from build123d import *

# Parameters (mm, degrees)
F1_DEPTH  = 330.2
F2_W      = 165.1
F2_H      = 35.56
F3_DEPTH  = 228.6
F4_SIZE   = 3.81
F6_DEPTH  = 25.4
F8_DEPTH  = 0.635
F9_DEPTH  = 25.4
F10_R     = 15.875
F11_DEPTH = 25.4
F12_SIZE  = 0.635


with BuildPart() as f1:
    # F0 (on Front) → F1 (new body)
    with BuildSketch(Plane.XZ):
        with BuildLine():
            Line((-76.581, 48.895), (-76.581, 0))
            Line((-76.581, 0), (76.581, 0))
            Line((76.581, 0), (76.581, 48.895))
            ThreePointArc((76.581, 48.895), (75.6510640303, 51.1400640303), (73.406, 52.07))
            Line((73.406, 52.07), (72.895141329, 52.07))
            ThreePointArc((72.895141329, 52.07), (70.8542906682, 51.3271911069), (69.7683767132, 49.4463329641))
            Line((69.7683767132, 49.4463329641), (63.3185122812, 12.8673340718))
            ThreePointArc((63.3185122812, 12.8673340718), (61.146684371, 9.1056177862), (57.0649830495, 7.62))
            Line((57.0649830495, 7.62), (0, 7.62))
            Line((0, 7.62), (-57.0649830495, 7.62))
            ThreePointArc((-57.0649830495, 7.62), (-61.146684371, 9.1056177862), (-63.3185122812, 12.8673340718))
            Line((-63.3185122812, 12.8673340718), (-69.7683767132, 49.4463329641))
            ThreePointArc((-69.7683767132, 49.4463329641), (-70.8542906682, 51.3271911069), (-72.895141329, 52.07))
            Line((-72.895141329, 52.07), (-73.406, 52.07))
            ThreePointArc((-73.406, 52.07), (-75.6510640303, 51.1400640303), (-76.581, 48.895))
        make_face()
    extrude(amount=F1_DEPTH)

    # F2 (on face) → F3 (cut)
    with BuildSketch(Plane.XZ.offset(330.2)):
        with Locations((0, 39.37)):
            Rectangle(F2_W, F2_H)
    extrude(amount=-F3_DEPTH, mode=Mode.SUBTRACT)

    # F4
    f4_edges = [f1.edges().sort_by_distance(p)[0] for p in [
        (76.581, -215.9, 21.59),
        (-76.581, -215.9, 21.59),
    ]]
    chamfer(f4_edges, length=F4_SIZE)

    # F5 (on face) → F6 (cut)
    with BuildSketch(Plane.XY.offset(7.62)):
        with BuildLine():
            Line((-57.9536338645, -28.1246478687), (-42.1049536604, -43.9733280728))
            ThreePointArc((-42.1049536604, -43.9733280728), (-53.0225, -76.2), (-42.1049536604, -108.4266719272))
            Line((-42.1049536604, -108.4266719272), (-57.9536338645, -124.2753521313))
            ThreePointArc((-57.9536338645, -124.2753521313), (-57.9536338645, -134.1536338645), (-48.0753521313, -134.1536338645))
            Line((-48.0753521313, -134.1536338645), (-32.2266719272, -118.3049536604))
            ThreePointArc((-32.2266719272, -118.3049536604), (0, -129.2225), (32.2266719272, -118.3049536604))
            Line((32.2266719272, -118.3049536604), (48.0753521313, -134.1536338645))
            ThreePointArc((48.0753521313, -134.1536338645), (57.9536338645, -134.1536338645), (57.9536338645, -124.2753521313))
            Line((57.9536338645, -124.2753521313), (42.1049536604, -108.4266719272))
            ThreePointArc((42.1049536604, -108.4266719272), (53.0225, -76.2), (42.1049536604, -43.9733280728))
            Line((42.1049536604, -43.9733280728), (57.9536338645, -28.1246478687))
            ThreePointArc((57.9536338645, -28.1246478687), (57.9536338645, -18.2463661355), (48.0753521313, -18.2463661355))
            Line((48.0753521313, -18.2463661355), (32.2266719272, -34.0950463396))
            ThreePointArc((32.2266719272, -34.0950463396), (0, -23.1775), (-32.2266719272, -34.0950463396))
            Line((-32.2266719272, -34.0950463396), (-48.0753521313, -18.2463661355))
            ThreePointArc((-48.0753521313, -18.2463661355), (-57.9536338645, -18.2463661355), (-57.9536338645, -28.1246478687))
        make_face()
    extrude(amount=-F6_DEPTH, mode=Mode.SUBTRACT)

    # F7 (on face) → F8 (cut)
    with BuildSketch(Plane.XY.offset(7.62)):
        with BuildLine():
            ThreePointArc((-60.1986978948, -30.3697118989), (-49.1264293251, -32.5721230524), (-42.8544929979, -23.1855070021))
            ThreePointArc((-42.8544929979, -23.1855070021), (-43.6278769476, -19.2974433292), (-45.8302881011, -16.0013021052))
            ThreePointArc((-45.8302881011, -16.0013021052), (-60.1986978948, -16.0013021052), (-60.1986978948, -30.3697118989))
        make_face()
        with BuildLine():
            ThreePointArc((-45.8302881011, -16.0013021052), (-43.6278769476, -19.2974433292), (-42.8544929979, -23.1855070021))
            ThreePointArc((-42.8544929979, -23.1855070021), (-49.1264293251, -32.5721230524), (-60.1986978948, -30.3697118989))
            Line((-60.1986978948, -30.3697118989), (-43.1340409794, -47.4343688143))
            Line((-43.1340409794, -47.4343688143), (-28.767801471, -33.0637887353))
            Line((-28.767801471, -33.0637887353), (-45.8302881011, -16.0013021052))
        make_face()
        with BuildLine():
            ThreePointArc((-45.8302881011, -136.3986978948), (-43.6278769476, -133.1025566708), (-42.8544929979, -129.2144929979))
            ThreePointArc((-42.8544929979, -129.2144929979), (-49.1264293251, -119.8278769476), (-60.1986978948, -122.0302881011))
            ThreePointArc((-60.1986978948, -122.0302881011), (-60.1986978948, -136.3986978948), (-45.8302881011, -136.3986978948))
        make_face()
        with BuildLine():
            ThreePointArc((-60.1986978948, -122.0302881011), (-49.1264293251, -119.8278769476), (-42.8544929979, -129.2144929979))
            ThreePointArc((-42.8544929979, -129.2144929979), (-43.6278769476, -133.1025566708), (-45.8302881011, -136.3986978948))
            Line((-45.8302881011, -136.3986978948), (-28.7656311857, -119.3340409794))
            Line((-28.7656311857, -119.3340409794), (-43.1362112647, -104.967801471))
            Line((-43.1362112647, -104.967801471), (-60.1986978948, -122.0302881011))
        make_face()
        with BuildLine():
            ThreePointArc((45.8302881011, -136.3986978948), (56.9025566708, -138.6011090482), (63.1744929979, -129.2144929979))
            ThreePointArc((63.1744929979, -129.2144929979), (62.4011090482, -125.3264293251), (60.1986978948, -122.0302881011))
            ThreePointArc((60.1986978948, -122.0302881011), (45.8302881011, -122.0302881011), (45.8302881011, -136.3986978948))
        make_face()
        with BuildLine():
            ThreePointArc((45.8302881011, -136.3986978948), (45.8302881011, -122.0302881011), (60.1986978948, -122.0302881011))
            Line((60.1986978948, -122.0302881011), (43.1340409794, -104.9656311857))
            Line((43.1340409794, -104.9656311857), (28.767801471, -119.3362112647))
            Line((28.767801471, -119.3362112647), (45.8302881011, -136.3986978948))
        make_face()
        with BuildLine():
            ThreePointArc((60.1986978948, -30.3697118989), (62.4011090482, -27.0735706749), (63.1744929979, -23.1855070021))
            ThreePointArc((63.1744929979, -23.1855070021), (56.9025566708, -13.7988909518), (45.8302881011, -16.0013021052))
            ThreePointArc((45.8302881011, -16.0013021052), (45.8302881011, -30.3697118989), (60.1986978948, -30.3697118989))
        make_face()
        with BuildLine():
            ThreePointArc((60.1986978948, -30.3697118989), (45.8302881011, -30.3697118989), (45.8302881011, -16.0013021052))
            Line((45.8302881011, -16.0013021052), (28.7656311857, -33.0659590206))
            Line((28.7656311857, -33.0659590206), (43.1362112647, -47.432198529))
            Line((43.1362112647, -47.432198529), (60.1986978948, -30.3697118989))
        make_face()
    extrude(amount=-F8_DEPTH, mode=Mode.SUBTRACT)

    # F7 (on face) → F9 (cut)
    with BuildSketch(Plane.XY.offset(7.62)):
        with BuildLine():
            ThreePointArc((-60.1986978948, -30.3697118989), (-49.1264293251, -32.5721230524), (-42.8544929979, -23.1855070021))
            ThreePointArc((-42.8544929979, -23.1855070021), (-43.6278769476, -19.2974433292), (-45.8302881011, -16.0013021052))
            ThreePointArc((-45.8302881011, -16.0013021052), (-60.1986978948, -16.0013021052), (-60.1986978948, -30.3697118989))
        make_face()
        with BuildLine():
            ThreePointArc((-45.8302881011, -16.0013021052), (-43.6278769476, -19.2974433292), (-42.8544929979, -23.1855070021))
            ThreePointArc((-42.8544929979, -23.1855070021), (-49.1264293251, -32.5721230524), (-60.1986978948, -30.3697118989))
            Line((-60.1986978948, -30.3697118989), (-43.1340409794, -47.4343688143))
            Line((-43.1340409794, -47.4343688143), (-28.767801471, -33.0637887353))
            Line((-28.767801471, -33.0637887353), (-45.8302881011, -16.0013021052))
        make_face()
        with BuildLine():
            ThreePointArc((-45.8302881011, -136.3986978948), (-43.6278769476, -133.1025566708), (-42.8544929979, -129.2144929979))
            ThreePointArc((-42.8544929979, -129.2144929979), (-49.1264293251, -119.8278769476), (-60.1986978948, -122.0302881011))
            ThreePointArc((-60.1986978948, -122.0302881011), (-60.1986978948, -136.3986978948), (-45.8302881011, -136.3986978948))
        make_face()
        with BuildLine():
            ThreePointArc((-60.1986978948, -122.0302881011), (-49.1264293251, -119.8278769476), (-42.8544929979, -129.2144929979))
            ThreePointArc((-42.8544929979, -129.2144929979), (-43.6278769476, -133.1025566708), (-45.8302881011, -136.3986978948))
            Line((-45.8302881011, -136.3986978948), (-28.7656311857, -119.3340409794))
            Line((-28.7656311857, -119.3340409794), (-43.1362112647, -104.967801471))
            Line((-43.1362112647, -104.967801471), (-60.1986978948, -122.0302881011))
        make_face()
        with BuildLine():
            ThreePointArc((45.8302881011, -136.3986978948), (56.9025566708, -138.6011090482), (63.1744929979, -129.2144929979))
            ThreePointArc((63.1744929979, -129.2144929979), (62.4011090482, -125.3264293251), (60.1986978948, -122.0302881011))
            ThreePointArc((60.1986978948, -122.0302881011), (45.8302881011, -122.0302881011), (45.8302881011, -136.3986978948))
        make_face()
        with BuildLine():
            ThreePointArc((45.8302881011, -136.3986978948), (45.8302881011, -122.0302881011), (60.1986978948, -122.0302881011))
            Line((60.1986978948, -122.0302881011), (43.1340409794, -104.9656311857))
            Line((43.1340409794, -104.9656311857), (28.767801471, -119.3362112647))
            Line((28.767801471, -119.3362112647), (45.8302881011, -136.3986978948))
        make_face()
        with BuildLine():
            ThreePointArc((60.1986978948, -30.3697118989), (62.4011090482, -27.0735706749), (63.1744929979, -23.1855070021))
            ThreePointArc((63.1744929979, -23.1855070021), (56.9025566708, -13.7988909518), (45.8302881011, -16.0013021052))
            ThreePointArc((45.8302881011, -16.0013021052), (45.8302881011, -30.3697118989), (60.1986978948, -30.3697118989))
        make_face()
        with BuildLine():
            ThreePointArc((60.1986978948, -30.3697118989), (45.8302881011, -30.3697118989), (45.8302881011, -16.0013021052))
            Line((45.8302881011, -16.0013021052), (28.7656311857, -33.0659590206))
            Line((28.7656311857, -33.0659590206), (43.1362112647, -47.432198529))
            Line((43.1362112647, -47.432198529), (60.1986978948, -30.3697118989))
        make_face()
    extrude(amount=F9_DEPTH, mode=Mode.SUBTRACT)

    # F10 (on face) → F11 (cut)
    with BuildSketch(Plane(origin=(0, 0, 0), x_dir=(1, 0, 0), z_dir=(0, 0, -1))):
        with Locations((0, 285.75)):
            Circle(F10_R)
        with Locations((0, 203.2)):
            Circle(F10_R)
    extrude(amount=-F11_DEPTH, mode=Mode.SUBTRACT)

    # F12
    f12_edges = [f1.edges().sort_by_distance(p)[0] for p in [
        (-15.875, -203.2, 7.62),
        (-15.875, -203.2, 0),
        (-15.875, -285.75, 0),
        (-15.875, -285.75, 7.62),
    ]]
    chamfer(f12_edges, length=F12_SIZE)


solid = f1.part
CAD build for the part. Positions are in the model's coordinates, mm. A direction names the side the tool comes from. Coordinates: 2 decimals unless noted, no trailing zeros. Order: outer loops, then holes, each group sorted by start corner. A loop starts at its lowest first (then second) coordinate and runs counter-clockwise, first axis right, second up. Notation, with made-up numbers: (-24.75, 42.25) -> (24.25, 42.25) arc R14 cw to (24.25, 56.25) -> close; hole circle Ø9 at (-0.5, 37). An arc over 180 degrees is marked (long way). Answer in a Markdown table with one row per item.
1) Drill centre lines: line 1 (X direction, y = -203, z = 3); line 2 (X direction, y = -144, z = 13); line 3 (Z direction, x = -1, y = -225). Where is each one in solid material? Low to high.
Check values:
| item | result |
|---|---|
| line 1 | -76.58 to -15.87, 15.87 to 76.58 |
| line 2 | -76.58 to -63.34, 63.34 to 76.58 |
| line 3 | 0 to 7.62 |
2) Which spindle directions (+Z, -Z, +X, -X, +Y, -Y) get a long thin tool onto all of the face, cutting with end or side? Do faces 1 (the face through (-63.153, -129.877, 8.408)), 2 (the face through (0.48, -23.18, 3.86)), 3 (the face through (-61.099, -162.789, 9.066)). Say none if no direction does.
Check values:
| item | result |
|---|---|
| face 1 | +Z |
| face 2 | +Z, -Z |
| face 3 | +Z, +Y, -Y |
3) Flat gauge pins, fed straight in: P1, Ø17, axis at x = 47.5, y = -125, coming from the +Z side (3 decimals); P2, Ø12, axis at x = 53.5, y = -123, coming from the +Z side; P3, Ø13, axis at x = -68.5, z = 37.5, coming from the -Y side. Where does each tip first touch, or does it go through?
Check values:
| item | result |
|---|---|
| P1 | z = 6.985 |
| P2 | z = 7.97 |
| P3 | y = -101.6 |
4) Band-saw the part on B-B (y = -203.2). List the corners of the cut face in (x, z) (3 decimals), and give its area (3 significant figures).
Check values:
| item | result |
|---|---|
| outline | (-76.581, 0) -> (-16.51, 0) -> (-15.875, 0.635) -> (-15.875, 6.985) -> (-16.51, 7.62) -> (-57.065, 7.62) arc R6.35 cw to (-63.319, 12.867) -> (-64.857, 21.59) -> (-72.771, 21.59) -> (-76.581, 17.78) -> close; (15.875, 0.635) -> (16.51, 0) -> (76.581, 0) -> (76.581, 17.78) -> (72.771, 21.59) -> (64.857, 21.59) -> (63.319, 12.867) arc R6.35 cw to (57.065, 7.62) -> (16.51, 7.62) -> (15.875, 6.985) -> close |
| area | 1,280 mm2 |
5) Band-saw the part on C-C (z = 42.5). List the corners of the cut face in (x, y), and give its area (3 significant figures).
Check values:
| item | result |
|---|---|
| outline | (-76.58, -101.6) -> (-68.54, -101.6) -> (-68.54, 0) -> (-76.58, 0) -> close; (68.54, -101.6) -> (76.58, -101.6) -> (76.58, 0) -> (68.54, 0) -> close |
| area | 1,630 mm2 |
6) Band-saw the part on A-A (x = 0). List the corners of the cut face in (y, z) (1 decimal), and give its area (3 significant figures).
Check values:
| item | result |
|---|---|
| outline | (-330.2, 0) -> (-302.3, 0) -> (-301.6, 0.6) -> (-301.6, 7) -> (-302.3, 7.6) -> (-330.2, 7.6) -> close; (-269.9, 0.6) -> (-269.2, 0) -> (-219.7, 0) -> (-219.1, 0.6) -> (-219.1, 7) -> (-219.7, 7.6) -> (-269.2, 7.6) -> (-269.9, 7) -> close; (-187.3, 0.6) -> (-186.7, 0) -> (-129.2, 0) -> (-129.2, 7.6) -> (-186.7, 7.6) -> (-187.3, 7) -> close; (-23.2, 0) -> (0, 0) -> (0, 7.6) -> (-23.2, 7.6) -> close |
| area | 1,220 mm2 |
7) Band-saw the part on D-D (y = -251). List the corners of the cut face in (x, z), and give its area (3 significant figures).
Check values:
| item | result |
|---|---|
| outline | (-76.58, 0) -> (76.58, 0) -> (76.58, 17.78) -> (72.77, 21.59) -> (64.86, 21.59) -> (63.32, 12.87) arc R6.35 cw to (57.06, 7.62) -> (-57.06, 7.62) arc R6.35 cw to (-63.32, 12.87) -> (-64.86, 21.59) -> (-72.77, 21.59) -> (-76.58, 17.78) -> close |
| area | 1,530 mm2 |
